```python
from build123d import *

# Parameters (mm, degrees)
BOSS_EXTRUDE1_DEPTH = 3.81
SKETCH2_R           = 4.458973568
BOSS_EXTRUDE2_DEPTH = 3.81
SKETCH3_R           = 2.437666758
CUT_EXTRUDE1_DEPTH  = 5.08
FILLET1_R           = 2.54
FILLET2_R           = 2.54


with BuildPart() as part:
    # Sketch1 → Boss-Extrude1 (new body)
    with BuildSketch(Plane.XY):
        Polygon((0, 30.495285818), (0, 36.722551391), (-33.610812147, 36.722551391), (-41.575749468, 9.669435316), (-43.362004736, 5.002722218), (-76.2, 5.002722218), (-76.2, 0), (-38.1, 0), (-29.121624295, 30.495285818), align=None)
    extrude(amount=BOSS_EXTRUDE1_DEPTH)

    # Sketch2 → Boss-Extrude2 (add)
    with BuildSketch(Plane.XY.offset(3.81)):
        with Locations((0, 33.608918604)):
            Circle(SKETCH2_R)
    extrude(amount=-BOSS_EXTRUDE2_DEPTH)

    # Sketch3 → Cut-Extrude1 (cut)
    with BuildSketch(Plane.XY.offset(3.81)):
        with Locations((0, 33.608918604)):
            Circle(SKETCH3_R)
    extrude(amount=-CUT_EXTRUDE1_DEPTH, mode=Mode.SUBTRACT)

    # Fillet1
    fillet1_edges = [part.edges().sort_by_distance(p)[0] for p in [
        (-33.610812147, 36.722551391, 1.905),
    ]]
    fillet(fillet1_edges, radius=FILLET1_R)

    # Fillet2
    fillet2_edges = [part.edges().sort_by_distance(p)[0] for p in [
        (-29.121624295, 30.495285818, 1.905),
    ]]
    fillet(fillet2_edges, radius=FILLET2_R)


solid = part.part
```
Could you check a few things on this model? Use its own coordinates, in mm. A direction names the side the tool comes from. Coordinates: 2 decimals unless noted, no trailing zeros. Write each loop counter-clockwise with the first axis right and the second up, starting at its lowest first coordinate (ties: lowest second). Pieces come first, ordered by that corner, then holes. Notation, with made-up numbers: M 60,45 L 117,45 A7 cw 117,54 Z; hole C 48,19 d1. An arc over 180 degrees is marked long. Answer as CSV lines item,"result". Start each with the question number.
1) Please list where these lines run through material, in increasing order: line 1 (Y direction, x = 0, z = 1.5); line 2 (Y direction, x = -24, z = 2.05); line 3 (X direction, y = 33, z = 0.55). Write a range as from..to.
2) I want a section at B-B, the plane z = 2.7. Please give me the cut outline in (x, y), and give its area (3 significant figures).
3) For faces 4 (the flat face through (-60, 5.003, 2)), 5 (the flat face through (-33, 21, 3.81)), 6 (the cylindrical face through (-28.725, 30.003, 1.932)), which set-ups out of +Z, -Z, +X, -X, +Y, -Y let a thin tool reach every point of the face, with its end or its side?
4) I want a section at D-D, the plane y = 20. Please give me the cut outline in (x, z).
5) We'd pull the mould along X, two halves only. Please class faces 1 (the flat face through (-33, 21, 0)), 2 (the cylindrical face through (-33.214, 36.23, 1.932)), 3 (the flat face through (-15, 30.495, 2)): +X half, -X half, draft (parallel to the pull), parting line (faces both ways), or undercut.
6) I want a section at A-A, the plane x = 0. Please give me the cut outline in (y, z).
7) For P1, Ø2, axis at x = -35, z = 0.5, coming from the +Y side; P2, Ø1.1, axis at x = -16, z = 1.5, coming from the +Y side, each with a flat end and sliding along its axis, tell me the tip position at first contact or that it passes through.
8) I want a section at C-C, the plane x = -52.5. Please give me the cut outline in (y, z), and give its area (3 significant figures).
Data:
1,line 1,"y = 29.15..31.17, 36.05..38.07"
1,line 2,"y = 30.5..36.72"
1,line 3,"x = -34.71..-2.36, 2.36..4.42"
2,outline,"M -76.2,0 L -38.1,0 L -29.66,28.67 A2.54 cw -27.22,30.5 L -3.19,30.5 A4.46 ccw long -3.19,36.72 L -31.71,36.72 A2.54 ccw -34.15,34.9 L -41.58,9.67 L -43.36,5 L -76.2,5 Z; hole C 0,33.61 d4.88"
2,area,"590 mm^2"
3,face 4,"+Z, -Z, -X, +Y"
3,face 5,"+Z, +X, -X, +Y, -Y"
3,face 6,"+Z, -Z, -Y"
4,outline,"M -38.53,0 L -32.21,0 L -32.21,3.81 L -38.53,3.81 Z"
5,face 1,"draft"
5,face 2,"-X half"
5,face 3,"undercut"
6,outline,"M 29.15,0 L 31.17,0 L 31.17,3.81 L 29.15,3.81 Z; M 36.05,0 L 38.07,0 L 38.07,3.81 L 36.05,3.81 Z"
7,P1,"stops at y = 35.28"
7,P2,"stops at y = 36.72"
8,outline,"M 0,0 L 5,0 L 5,3.81 L 0,3.81 Z"
8,area,"19.1 mm^2"
